```python
from build123d import *

# Parameters (mm, degrees)
SKETCH009_W             = 84
SKETCH009_H             = 70
PAD002_DEPTH            = 2
SKETCH010_W             = 2
SKETCH010_H             = 7
PAD003_DEPTH            = 2
SKETCH012_W             = 8
SKETCH012_H             = 6.8
PAD004_DEPTH            = 4
SKETCH013_W             = 7
SKETCH013_H             = 6
PAD005_DEPTH            = 4
SKETCH011_W             = 8
SKETCH011_H             = 6.8
PAD006_DEPTH            = 4
SKETCH014_R             = 1.15
POCKET002_DEPTH         = 81.001
SKETCH016_R             = 1.15
POCKET003_DEPTH         = 8.501
SKETCH018_W             = 11.5
SKETCH018_H             = 11.5
POCKET004_DEPTH         = 5
POCKET005_DEPTH         = 5
POCKET006_DEPTH         = 5
SKETCH021_W             = 1
SKETCH021_H             = 7
PAD007_DEPTH            = 1
SKETCH022_W             = 9
SKETCH022_H             = 10
POCKET007_DEPTH         = 0.4
FILLET_R                = 3
BODY002_PITCH_ANGLE     = -90
BODY002_PLACEMENT_ANGLE = 90
PAD001_DEPTH            = 42
SKETCH007_W             = 11.5
SKETCH007_H             = 11.5
POCKET001_DEPTH         = 13
FILLET001_R             = 3
SKETCH025_W             = 6.5
SKETCH025_H             = 9
SKETCH025_W_2           = 9
SKETCH025_H_2           = 6.5
POCKET008_DEPTH         = 3.5


with BuildPart() as back:
    # Sketch009 → Pad002 (new body)
    with BuildSketch(Plane.XY):
        Rectangle(SKETCH009_W, SKETCH009_H)
    extrude(amount=PAD002_DEPTH)

    # Sketch010 (on Face6 of Pad002) → Pad003 (join)
    with BuildSketch(Plane.XY.offset(2)):
        with Locations((-38, -1)):
            Rectangle(SKETCH010_W, SKETCH010_H)
        Polygon((-21, 32), (39, 32), (39, -4), (37, -4), (37, 30), (-21, 30), align=None)
    extrude(amount=PAD003_DEPTH)

    # Sketch012 (on Face15 of Pad003) → Pad004 (join)
    with BuildSketch(Plane.YZ.offset(39)):
        with Locations((0, 5.4)):
            Rectangle(SKETCH012_W, SKETCH012_H)
    extrude(amount=-PAD004_DEPTH)

    # Sketch013 (on Face9 of Pad004) → Pad005 (join)
    with BuildSketch(Plane(origin=(-39, 0, 0), x_dir=(0, -1, 0), z_dir=(-1, 0, 0))):
        with Locations((1, 5)):
            Rectangle(SKETCH013_W, SKETCH013_H)
    extrude(amount=-PAD005_DEPTH)

    # Sketch011 (on Face16 of Pad003) → Pad006 (join)
    with BuildSketch(Plane(origin=(0, 32, 0), x_dir=(-1, 0, 0), z_dir=(0, 1, 0))):
        with Locations((-29, 5.4)):
            Rectangle(SKETCH011_W, SKETCH011_H)
        with Locations((14, 5.4)):
            Rectangle(SKETCH011_W, SKETCH011_H)
    extrude(amount=-PAD006_DEPTH)

    # Sketch014 (on Face44 of Pad006) → Pocket002 (cut, through all)
    with BuildSketch(Plane.YZ.offset(39)):
        with Locations((0, 5)):
            Circle(SKETCH014_R)
    extrude(amount=-POCKET002_DEPTH, mode=Mode.SUBTRACT)

    # Sketch016 → Pocket003 (cut, through all)
    with BuildSketch(Plane.XZ.offset(-26.5)):
        with Locations((-13, 5)):
            Circle(SKETCH016_R)
        with Locations((30, 5)):
            Circle(SKETCH016_R)
    extrude(amount=-POCKET003_DEPTH, mode=Mode.SUBTRACT)

    # Sketch018 (on Face5 of Pocket003) → Pocket004 (cut)
    with BuildSketch(Plane.XY.offset(2)):
        with Locations((0, 17.75)):
            Rectangle(SKETCH018_W, SKETCH018_H)
    extrude(amount=-POCKET004_DEPTH, mode=Mode.SUBTRACT)

    # Sketch019 (on Face31 of Pocket004) → Pocket005 (cut)
    with BuildSketch(Plane.XZ.offset(-28)):
        Polygon((29.125944, 9.042901), (33.258869, 4.499726), (33.258869, 9.042901), align=None)
    extrude(amount=-POCKET005_DEPTH, mode=Mode.SUBTRACT)

    # Sketch020 (on Face36 of Pocket005) → Pocket006 (cut)
    with BuildSketch(Plane(origin=(35, 0, 0), x_dir=(0, -1, 0), z_dir=(-1, 0, 0))):
        Polygon((2.77547, 8.938441), (6.386171, 3.079567), (6.386171, 8.938441), align=None)
    extrude(amount=-POCKET006_DEPTH, mode=Mode.SUBTRACT)

    # Sketch021 (on Face40 of Pocket006) → Pad007 (join)
    with BuildSketch(Plane.XY.offset(8)):
        with Locations((-38.5, -1)):
            Rectangle(SKETCH021_W, SKETCH021_H)
    extrude(amount=PAD007_DEPTH)

    # Sketch022 (on Face5 of Pocket005) → Pocket007 (cut)
    with BuildSketch(Plane.XY.offset(2)):
        with Locations((-30.3, 30)):
            Rectangle(SKETCH022_W, SKETCH022_H)
    extrude(amount=-POCKET007_DEPTH, mode=Mode.SUBTRACT)

    # Fillet
    fillet_edges = [back.edges().sort_by_distance(p)[0] for p in [
        (42, 35, 1),
        (-42, 35, 1),
    ]]
    fillet(fillet_edges, radius=FILLET_R)


with BuildPart() as back_1:
    # Body002 pitch: moved
    add(back.part.rotate(Axis((0, 0, 0), (0, 1, 0)), BODY002_PITCH_ANGLE))


with BuildPart() as back_2:
    # Body002 placement: moved
    add(back_1.part.rotate(Axis((0, 0, 0), (0, 0, 1)), BODY002_PLACEMENT_ANGLE))


with BuildPart() as curve:
    # Sketch006 → Pad001 (new body, symmetric)
    with BuildSketch(Plane.XY):
        with BuildLine():
            ThreePointArc((-35, 1.796592), (0.104214, 0.997658), (35, 4.9))
            Line((35, -0.1), (35, 4.9))
            Line((-35, -0.1), (35, -0.1))
            Line((-35, 1.796592), (-35, -0.1))
        make_face()
    extrude(amount=PAD001_DEPTH, both=True)

    # Sketch007 (on Face3 of Pad001) → Pocket001 (cut)
    with BuildSketch(Plane.XZ.offset(0.1)):
        with Locations((-17.75, 0)):
            Rectangle(SKETCH007_W, SKETCH007_H)
    extrude(amount=-POCKET001_DEPTH, mode=Mode.SUBTRACT)

    # Fillet001
    fillet001_edges = [curve.edges().sort_by_distance(p)[0] for p in [
        (-35, 0.848296, -42),
        (-35, 0.848296, 42),
    ]]
    fillet(fillet001_edges, radius=FILLET001_R)

    # Boolean: union Back
    add(back_2.part)

    # Sketch025 (on Face32 of Boolean) → Pocket008 (cut, symmetric)
    with BuildSketch(Plane.XZ.offset(2)):
        with Locations((-28.75, 0)):
            Rectangle(SKETCH025_W, SKETCH025_H)
        with Locations((-15.55, 13.625)):
            Rectangle(SKETCH025_W_2, SKETCH025_H_2)
        with Locations((-2.05, 0)):
            Rectangle(SKETCH025_W, SKETCH025_H)
        with Locations((-15.55, -13.625)):
            Rectangle(SKETCH025_W_2, SKETCH025_H_2)
    extrude(amount=POCKET008_DEPTH, both=True, mode=Mode.SUBTRACT)


solid = curve.part
```
The listing builds one solid part. Answer for the finished solid, in the listing's coordinates (mm). A direction names the side the tool comes from. Give positions to 0.01 mm unless a question says otherwise; leave off trailing zeros. Order: outer loops, then holes, each group sorted by start corner. A loop starts at its lowest first (then second) coordinate and runs counter-clockwise, first axis right, second up. Notation, with made-up numbers: M 58.5,-7 L 92.5,-7 A19 ccw 92.5,21 Z; hole C -14.75,-10.75 d3. An arc over 180 degrees is marked long. Put each result on its own line as item: value. Start each with the question number.
Item 1: The part is cut by section C-C, the plane x = -27. Determine the outline of the cut face in (y, z).
Item 2: The part is cut by section B-B, the plane x = 0. Determine the outline of the cut face in (y, z), and give its area (3 significant figures).
Item 3: For a pull along Z with two mould halves and no side action, classify faces 5 (the face through (-34.1, -0.13, -41.14)), 6 (the face through (35, 1, -1)), 7 (the face through (-23.5, -1, 0)) as +Z half, -Z half, draft (parallel to the pull), parting line (faces both ways), or undercut.
Item 4: Flat-ended cylindrical pins translate along their axes: P1, Ø2, axis at y = -6, z = -36.5, coming from the +X side; P2, Ø4, axis at x = -18, z = -24.5, coming from the -Y side; P3, Ø5, axis at y = 2.5, z = -27.5, coming from the -X side; P4, Ø12, axis at x = -9.5, z = -16.5, coming from the +Y side. Find the tip coordinate at first contact, or state that the pin passes through.
Item 5: Find the intervals of material crossed by line 1 along Y through (x, z) = (0, -37); line 2 along Z through (x, y) = (-28, -0.75); line 3 along Z through (x, y) = (1.5, -6.5), in increasing order.
Item 6: The part is cut by section A-A, the plane z = -13. Determine the outline of the cut face in (x, y), and give its area (3 significant figures).
Item 7: The part is cut by section D-D, the plane z = -31.5. Determine the outline of the cut face in (x, y), and give its area (3 significant figures).
Item 8: Which of the six approach directions +Z, -Z, +X, -X, +Y, -Y give full straight-line access (tool end or side, diameter ignored) to faces 1 (the face through (-30, -3, 35)), 2 (the face through (4, -4, 37)), 3 (the face through (-16, -1, -16.875)), 4 (the face through (-31, -3, -21))?
Answer key:
1. outline: M -4,37 L -2,37 L -2,4.5 L 1.2,4.5 L 1.2,42 L -2,42 L -2,39 L -4,39 Z; M -2,-42 L 1.2,-42 L 1.2,-4.5 L -2,-4.5 L -2,-25.8 L -1.6,-25.8 L -1.6,-34.8 L -2,-34.8 Z
2. outline: M -9,-39 L -6.15,-39 L -6.15,-35 L -8,-35 L -8,-38 L -9,-38 Z; M -8.8,35 L -6.15,35 L -6.15,39 L -8.8,39 Z; M -3.85,-39 L -2,-39 L -2,-42 L 0.99,-42 L 0.99,-4.5 L -2,-4.5 L -2,-35 L -3.85,-35 Z; M -3.85,35 L -2,35 L -2,4.5 L 0.99,4.5 L 0.99,42 L -2,42 L -2,39 L -3.85,39 Z
2. area: 258 mm²
3. face 5: -Z half
3. face 6: draft
3. face 7: undercut
4. P1: stops at x = 4.5
4. P2: stops at y = -2
4. P3: stops at x = -35
4. P4: stops at y = 0.86
5. line 1: y = -8 to -6.15, -3.85 to 0.99
5. line 2: z = -42 to -4.5, 4.5 to 42
5. line 3: z = -39 to -35, 35 to 39
6. outline: M -35,-2 L -32,-2 L -32,-3.85 L -28,-3.85 L -28,-2 L -20.05,-2 L -20.05,0.88 A262 cw -35,1.8 Z; M -32,-8.8 L -28,-8.8 L -28,-6.15 L -32,-6.15 Z; M -11.05,-2 L 35,-2 L 35,4.9 A262 cw -11.05,0.74 Z
6. area: 257 mm²
7. outline: M -35,-1.6 L -25,-1.6 L -25,-2 L 35,-2 L 35,4.9 A262 cw -35,1.8 Z
7. area: 260 mm²
8. face 1: -Y
8. face 2: +Z, +X, -Y
8. face 3: +Y, -Y
8. face 4: -Z, +X, -X, -Y
